Read the model definition and answer for the solid it produces. Units are mm, in the model's axes. A direction names the side the tool comes from. Coordinates: 2 decimals unless noted, no trailing zeros. Loops run counter-clockwise (first coordinate to the right, second up) from the corner with the lowest first, then second, coordinate; pieces in that order, holes last. Notation, with made-up numbers: (8.25, 17) -> (17.25, 17) arc R20 cw to (17.25, 54) -> close; hole circle Ø6 at (24.5, -13). An arc over 180 degrees is marked (long way). Answer as CSV lines item,"result".
```python
from build123d import *

# Parameters (mm, degrees)
SKETCH1_W           = 50
SKETCH1_H           = 30
BOSS_EXTRUDE1_DEPTH = 10
CUT_EXTRUDE1_DEPTH  = 5
SKETCH3_R           = 2.6
CUT_EXTRUDE2_DEPTH  = 451.671399096
FILLET1_R           = 10


with BuildPart() as part:
    # Sketch1 → Boss-Extrude1 (new body)
    with BuildSketch(Plane.XY):
        with Locations((0, 434.949674923)):
            Rectangle(SKETCH1_W, SKETCH1_H)
    extrude(amount=BOSS_EXTRUDE1_DEPTH)

    # Sketch2 → Cut-Extrude1 (cut)
    with BuildSketch(Plane(origin=(0, 0, 0), x_dir=(-1, 0, 0), z_dir=(0, 0, -1))):
        Polygon((11, 430.259075999), (15, 432.568477076), (19, 430.259075999), (19, 425.640273846), (15, 423.330872769), (11, 425.640273846), align=None)
        Polygon((-15, 432.568477076), (-19, 430.259075999), (-19, 425.640273846), (-15, 423.330872769), (-11, 425.640273846), (-11, 430.259075999), align=None)
    extrude(amount=-CUT_EXTRUDE1_DEPTH, mode=Mode.SUBTRACT)

    # Sketch3 → Cut-Extrude2 (cut, through all)
    with BuildSketch(Plane(origin=(0, 0, 5), x_dir=(-1, 0, 0), z_dir=(0, 0, -1))):
        with Locations((15, 427.949674923)):
            Circle(SKETCH3_R)
        with Locations(Location((-15, 427.949674923, 0), (0, 0, 180))):
            Circle(SKETCH3_R)
    extrude(amount=-CUT_EXTRUDE2_DEPTH, mode=Mode.SUBTRACT)

    # Fillet1
    fillet1_edges = [part.edges().sort_by_distance(p)[0] for p in [
        (25, 419.949674923, 5),
        (-25, 419.949674923, 5),
    ]]
    fillet(fillet1_edges, radius=FILLET1_R)


solid = part.part
```
Q1. For faces 4 (the face through (-16.97, 431.43, 2.46)), 5 (the face through (21.99, 422.8, 5.07)), determine the directions among +Z, -Z, +X, -X, +Y, -Y from which every point of the face is accessible in a straight line to the end or side of a thin tool.
Results:
face 4,"-Z"
face 5,"+Z, -Z, +X, -Y"
Q2. For a pull along Y with two mould halves and no side action, classify faces 1 (the face through (0, 419.95, 5)), 2 (the face through (0, 435, 10)), 3 (the face through (-14.662, 430.528, 7.465)) as pulls with the +Y half, pulls with the -Y half, needs draft (parallel to the pull), parting line crosses it, or undercut.
Results:
face 1,"pulls with the -Y half"
face 2,"needs draft"
face 3,"undercut"
Q3. Given pin 1 Ø1.5 at (x, y) = (3.5, 446) entering from -Z; pin 2 Ø2.5 at (y, z) = (428, 2.5) entering from +X; pin 3 Ø2.5 at (x, y) = (16.5, 426) entering from -Z; pin 4 Ø3.5 at (y, z) = (427.5, 2.5) entering from -X, each flat-ended and moving along its own axis, determine where each tip first touches the part or whether it passes through.
Results:
pin 1,"stops at z = 0"
pin 2,"stops at x = 24.98"
pin 3,"stops at z = 5"
pin 4,"stops at x = -24.98"
Q4. A cutting plane is placed at B-B, the plane z = 9. Write down the section's boundary in (x, y), and give its area (3 significant figures).
Results:
outline,"(-25, 429.95) arc R10 ccw to (-15, 419.95) -> (15, 419.95) arc R10 ccw to (25, 429.95) -> (25, 449.95) -> (-25, 449.95) -> close; hole circle Ø5.2 at (-15, 427.95); hole circle Ø5.2 at (15, 427.95)"
area,"1,410 mm²"
Q5. Find the intervals of material crossed by probe 1 along X at (y, z) = (427.5, 9.25); probe 2 along X at (y, z) = (430.75, 3.25); probe 3 along Y at (x, z) = (-15, 6), in increasing order. Write a range as [from, to].
Results:
probe 1,"x = [-24.7, -17.56], [-12.44, 12.44], [17.56, 24.7]"
probe 2,"x = [-25, -18.15], [-11.85, 11.85], [18.15, 25]"
probe 3,"y = [419.95, 425.35], [430.55, 449.95]"
Q6. A cutting plane is placed at A-A, the plane z = 3.75. Write down the section's boundary in (x, y), and give its area (3 significant figures).
Results:
outline,"(-25, 429.95) arc R10 ccw to (-15, 419.95) -> (15, 419.95) arc R10 ccw to (25, 429.95) -> (25, 449.95) -> (-25, 449.95) -> close; hole (-19, 425.64) -> (-15, 423.33) -> (-11, 425.64) -> (-11, 430.26) -> (-15, 432.57) -> (-19, 430.26) -> close; hole (11, 425.64) -> (15, 423.33) -> (19, 425.64) -> (19, 430.26) -> (15, 432.57) -> (11, 430.26) -> close"
area,"1,350 mm²"
Q7. A cutting plane is placed at C-C, the plane y = 422. Write down the section's boundary in (x, z), and give its area (3 significant figures).
Results:
outline,"(-21.07, 0) -> (21.07, 0) -> (21.07, 10) -> (-21.07, 10) -> close"
area,"421 mm²"
